from build123d import *

# Parameters (mm, degrees)
F0_W     = 85.725
F0_H     = 69.2404
F1_DEPTH = 9.525
F2_T     = -4.7498
F3_R     = 0.635
F4_DEPTH = 4.7625
F5_R     = 2.286


with BuildPart() as f1:
    # F0 (on Top) → F1 (new body)
    with BuildSketch(Plane.XY):
        Rectangle(F0_W, F0_H)
    extrude(amount=F1_DEPTH)

    # F2
    f2_openings = [f1.faces().sort_by_distance(p)[0] for p in [
        (0, 0, 9.525),
    ]]
    offset(amount=F2_T, openings=f2_openings)

    # F3 (on face) → F4 (cut)
    with BuildSketch(Plane.XY.offset(9.525)):
        with Locations((-38.1127, 29.8704)):
            Circle(F3_R)
        with Locations((38.1127, 29.8704)):
            Circle(F3_R)
        with Locations((38.1127, -29.8704)):
            Circle(F3_R)
        with Locations((-38.1127, -29.8704)):
            Circle(F3_R)
    extrude(amount=-F4_DEPTH, mode=Mode.SUBTRACT)

    # F5
    f5_edges = [f1.edges().sort_by_distance(p)[0] for p in [
        (0, -34.6202, 9.525),
        (-42.8625, -34.6202, 4.7625),
        (-42.8625, 0, 0),
        (-42.8625, 0, 9.525),
        (0, -34.6202, 0),
        (42.8625, -34.6202, 4.7625),
        (-42.8625, 34.6202, 4.7625),
        (0, 34.6202, 9.525),
        (0, 34.6202, 0),
        (42.8625, 34.6202, 4.7625),
        (42.8625, 0, 9.525),
        (42.8625, 0, 0),
    ]]
    fillet(f5_edges, radius=F5_R)


solid = f1.part
Model file for the job. Use its own axes, mm. A direction names the side the tool comes from. Give positions to 0.01 mm unless a question says otherwise; leave off trailing zeros. Write each loop counter-clockwise with the first axis right and the second up, starting at its lowest first coordinate (ties: lowest second). Pieces come first, ordered by that corner, then holes. Notation, with made-up numbers: (45.25, -14.75) - (104.25, -14.75) arc R16 cw to (104.25, 7.25) - close; hole circle Ø8 at (9.5, 70.5). An arc over 180 degrees is marked (long way). Answer as CSV lines item,"result".
1. Band-saw the part on A-A (x = -18). Write the cut outline in (y, z) (3 decimals), and give its area (3 significant figures).
Responses:
outline,"(-34.62, 2.286) arc R2.286 ccw to (-32.334, 0) - (32.334, 0) arc R2.286 ccw to (34.62, 2.286) - (34.62, 7.239) arc R2.286 ccw to (32.334, 9.525) - (29.87, 9.525) - (29.87, 4.75) - (-29.87, 4.75) - (-29.87, 9.525) - (-32.334, 9.525) arc R2.286 ccw to (-34.62, 7.239) - close"
area,"370 mm2"
2. Pin check, flat tips, straight feed: pin 1 (1.4 mm diameter, centred on y = -7, z = 7.5, fed in from +X); pin 2 (3 mm diameter, centred on x = -13.5, y = -6, fed in from +Z). Stop position of each tip, or through.
Responses:
pin 1,"stops at x = 42.86"
pin 2,"stops at z = 4.75"
3. Drill centre lines: L1, parallel to Y at x = -29, z = 7; L2, parallel to X at y = -9, z = 7; L3, parallel to X at y = 30, z = 8. Where is each one in solid material? Low to high. Write a range as [from, to].
Responses:
L1,"y = [-34.62, -29.87], [29.87, 34.62]"
L2,"x = [-42.86, -38.11], [38.11, 42.86]"
L3,"x = [-42.73, -38.73], [-37.49, 37.49], [38.73, 42.73]"
4. Band-saw the part on B-B (z = 5.75). Write the cut outline in (x, y) (1 decimal).
Responses:
outline,"(-42.9, -32.3) arc R2.3 ccw to (-40.6, -34.6) - (40.6, -34.6) arc R2.3 ccw to (42.9, -32.3) - (42.9, 32.3) arc R2.3 ccw to (40.6, 34.6) - (-40.6, 34.6) arc R2.3 ccw to (-42.9, 32.3) - close; hole (-38.1, -29.2) arc R0.6 ccw (long way) to (-37.5, -29.9) - (37.5, -29.9) arc R0.6 ccw (long way) to (38.1, -29.2) - (38.1, 29.2) arc R0.6 ccw (long way) to (37.5, 29.9) - (-37.5, 29.9) arc R0.6 ccw (long way) to (-38.1, 29.2) - close"
5. 3-axis set-ups, long thin cutter, end or side, ignore diameter. For faces 1 (the face through (42.862, 0, 5)), 2 (the face through (-1, -29.87, 7)): which of +Z, -Z, +X, -X, +Y, -Y reach the whole face in a straight line?
Responses:
face 1,"+Z, -Z, +X, +Y, -Y"
face 2,"+Z"
6. Band-saw the part on C-C (y = 7). Write the cut outline in (x, z) (1 decimal), and give its area (3 significant figures).
Responses:
outline,"(-42.9, 2.3) arc R2.3 ccw to (-40.6, 0) - (40.6, 0) arc R2.3 ccw to (42.9, 2.3) - (42.9, 7.2) arc R2.3 ccw to (40.6, 9.5) - (38.1, 9.5) - (38.1, 4.7) - (-38.1, 4.7) - (-38.1, 9.5) - (-40.6, 9.5) arc R2.3 ccw to (-42.9, 7.2) - close"
area,"448 mm2"
